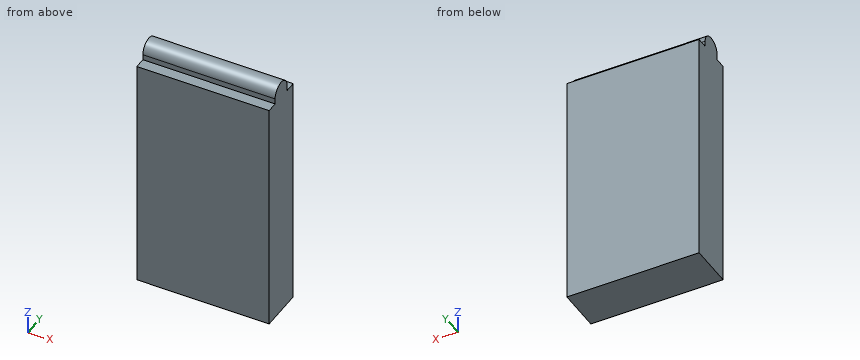
```python
from build123d import *

# Parameters (mm, degrees)
SKETCH_1_W      = 24
SKETCH_1_H      = 43
EXTRUDE_1_DEPTH = 8
EXTRUDE_2_DEPTH = 24


with BuildPart() as part:
    # 草图1 → 凸台-拉伸1 (new body)
    with BuildSketch(Plane(origin=(0, 0, 0), x_dir=(1, 0, 0), z_dir=(0, 1, 0))):
        with Locations((12, 21.5)):
            Rectangle(SKETCH_1_W, SKETCH_1_H)
    extrude(amount=EXTRUDE_1_DEPTH)

    # 草图2 → 凸台-拉伸2 (add)
    with BuildSketch(Plane(origin=(24, 0, 0), x_dir=(0, 0, -1), z_dir=(1, 0, 0))):
        with BuildLine():
            Line((0, 2), (-1, 2))
            ThreePointArc((-1, 2), (-3, 4), (-1, 6))
            Line((-1, 6), (0, 6))
            ThreePointArc((0, 6), (2, 4), (0, 2))
        make_face()
    extrude(amount=-EXTRUDE_2_DEPTH)


solid = part.part
```
CAD build for the part. Positions are in the model's coordinates, mm. Round coordinates to 2 decimals unless told otherwise and drop trailing zeros. Loops run counter-clockwise (first coordinate to the right, second up) from the corner with the lowest first, then second, coordinate; pieces in that order, holes last. Notation, with made-up numbers: M 68,52.5 L 116,52.5 A18 cw 116,67.5 Z; hole C 23.5,3.25 d1. An arc over 180 degrees is marked long. Use a Markdown table: item, result. Add a question column.
(1) Cut at A-A (x = 16). Give the cut face in (y, z), and give its area (3 significant figures).
(2) Flat gauge pins, fed straight in: pin 1 (0.6 mm diameter, centred on x = 10.5, y = 1, fed in from +Z); pin 2 (0.8 mm diameter, centred on x = 7, z = 0.5, fed in from +Y). Where does each tip first touch, or does it go through?
(3) Drill centre lines: line 1 (Z direction, x = 16, y = 7.5); line 2 (Z direction, x = 18.75, y = 4.25). Where is each one in solid material? Low to high.
(4) Cut at B-B (y = 1). Give the cut face in (x, z).
Geometry says:
| question | item | result |
|---|---|---|
| 1 | outline | M 0,-43 L 8,-43 L 8,0 L 6,0 L 6,1 A2 ccw 2,1 L 2,0 L 0,0 Z |
| 1 | area | 354 mm² |
| 2 | pin 1 | stops at z = 0 |
| 2 | pin 2 | stops at y = 6 |
| 3 | line 1 | z = -43 to 0 |
| 3 | line 2 | z = -43 to 2.98 |
| 4 | outline | M 0,-43 L 24,-43 L 24,0 L 0,0 Z |
